The model under review builds one solid part; all positions refer to its coordinate system, in mm. Coordinates: 2 decimals unless noted, no trailing zeros. Order: outer loops, then holes, each group sorted by start corner. A loop starts at its lowest first (then second) coordinate and runs counter-clockwise, first axis right, second up. Notation, with made-up numbers: (61, 5.5) -> (111, 5.5) arc R24 ccw to (111, 26.5) -> close; hole circle Ø1 at (-36, -26.75). An arc over 180 degrees is marked (long way). Use one line per item in the form item = value.
from build123d import *

# Parameters (mm, degrees)
SKETCH1_W                     = 1
SKETCH1_H                     = 102
REVOLVE_THIN1_ANGLE           = 15
REVOLVE_THIN1_OTHER_WAY_ANGLE = 165
F_4_5_4_5_DIAMETER_HOLE1_D    = 4.5
CIRPATTERN1_COUNT             = 12
F_4_0_4_DIAMETER_HOLE1_D      = 4
CIRPATTERN2_COUNT             = 4
F_4_5_4_5_DIAMETER_HOLE2_D    = 4.5
CIRPATTERN3_COUNT             = 2
CIRPATTERN3_ANGLE             = 90
CUT_EXTRUDE1_DEPTH            = 2
CUT_EXTRUDE2_DEPTH            = 2
FILLET1_R                     = 1


with BuildPart() as part:
    # Sketch1 → Revolve-Thin1 (revolve)
    with BuildSketch(Plane(origin=(0, 0, 0), x_dir=(0, 0, -1), z_dir=(1, 0, 0))):
        with Locations((-0.5, 80)):
            Rectangle(SKETCH1_W, SKETCH1_H)
    revolve(axis=Axis((0, 0, 0), (0, 0, 1)), revolution_arc=REVOLVE_THIN1_ANGLE)

    # Sketch1 → Revolve-Thin1 other way (revolve)
    with BuildSketch(Plane(origin=(0, 0, 0), x_dir=(0, 0, -1), z_dir=(1, 0, 0))):
        with Locations((-0.5, 80)):
            Rectangle(SKETCH1_W, SKETCH1_H)
    revolve(axis=Axis((0, 0, 0), (0, 0, -1)), revolution_arc=REVOLVE_THIN1_OTHER_WAY_ANGLE)

    # Ø4.5 (4.5) Diameter Hole1 (through all)
    with Locations(Plane.XY.offset(1)):
        with Locations((62.125, 107.60365642)):
            f_4_5_4_5_diameter_hole1 = Hole(F_4_5_4_5_DIAMETER_HOLE1_D / 2)

    # CirPattern1: Ø4.5 (4.5) Diameter Hole1 ×12 about axis, 8 skipped
    cirpattern1_axis = Axis((0, 0, -80.9), (0, 0, 1))
    add([f_4_5_4_5_diameter_hole1.rotate(cirpattern1_axis, i * 360 / CIRPATTERN1_COUNT) for i in range(1, CIRPATTERN1_COUNT) if i not in (1, 2, 3, 4, 5, 6, 7, 10)], mode=Mode.SUBTRACT)

    # Ø4.0 (4) Diameter Hole1 (through all)
    with Locations(Plane.XY.offset(1)):
        with Locations((124.25, 0)):
            f_4_0_4_diameter_hole1 = Hole(F_4_0_4_DIAMETER_HOLE1_D / 2)

    # CirPattern2: Ø4.0 (4) Diameter Hole1 ×4 about axis, 2 skipped
    cirpattern2_axis = Axis((0, 0, -80.9), (0, 0, 1))
    add([f_4_0_4_diameter_hole1.rotate(cirpattern2_axis, i * 360 / CIRPATTERN2_COUNT) for i in range(1, CIRPATTERN2_COUNT) if i not in (2, 3)], mode=Mode.SUBTRACT)

    # Ø4.5 (4.5) Diameter Hole2 (through all)
    with Locations(Plane.XY.offset(1)):
        with Locations((87.858017562, 87.858017562)):
            f_4_5_4_5_diameter_hole2 = Hole(F_4_5_4_5_DIAMETER_HOLE2_D / 2)

    # CirPattern3: Ø4.5 (4.5) Diameter Hole2 ×2 about axis
    cirpattern3_axis = Axis((0, 0, -80.9), (0, 0, -1))
    for i in range(1, CIRPATTERN3_COUNT):
        add(f_4_5_4_5_diameter_hole2.rotate(cirpattern3_axis, i * CIRPATTERN3_ANGLE / (CIRPATTERN3_COUNT - 1)), mode=Mode.SUBTRACT)

    # Sketch12 → Cut-Extrude1 (cut, through all)
    with BuildSketch(Plane.XY.offset(1)):
        with BuildLine():
            Line((0.707106781, 126.371320344), (2.121320344, 124.957106781))
            ThreePointArc((2.121320344, 124.957106781), (2.121320344, 122.128679656), (-0.707106781, 122.128679656))
            Line((-0.707106781, 122.128679656), (-2.121320344, 123.542893219))
            ThreePointArc((-2.121320344, 123.542893219), (-2.121320344, 126.371320344), (0.707106781, 126.371320344))
        make_face()
    extrude(amount=-CUT_EXTRUDE1_DEPTH, mode=Mode.SUBTRACT)

    # Sketch13 → Cut-Extrude2 (cut, through all)
    with BuildSketch(Plane.XY.offset(1)):
        Polygon((-33.905294908, 126.536283244), (33.905294908, -126.536283244), (34.001887491, -126.510401339), (-33.808702326, 126.562165148), align=None)
    extrude(amount=-CUT_EXTRUDE2_DEPTH, mode=Mode.SUBTRACT)

    # Fillet1
    fillet1_edges = [part.edges().sort_by_distance(p)[0] for p in [
        (-7.409115101, 28.037564327, 0.5),
        (7.602300266, -27.985800518, 0.5),
        (34.001877612, -126.510364472, 0.5),
        (-33.808692447, 126.562128281, 0.5),
    ]]
    fillet(fillet1_edges, radius=FILLET1_R)


solid = part.part
Item 1: We need section A-A (z = 0.6). State how many separate pieces and enclosed holes the cut face has, plus the area to 3 significant figures.
Results found:
separate_pieces = 1
enclosed_holes = 8
area = 25,500 mm²
Item 2: Draft analysis for pull direction Y (two halves, no side actions). For faces 1 (the face through (50, 4, 0)), 2 (the face through (125.764, 36.665, 0.493)), 3 (the face through (27.844, 8.106, 0.493)), state which applies: released by +Y, released by -Y, zero draft, split by the parting line, or undercut.
Results found:
face_1 = zero draft
face_2 = split by the parting line
face_3 = undercut
Item 3: To check wall thickness, follow L1, parallel to Y at x = 109.5, z = 0.45; L2, parallel to Y at x = -1, z = 0.35; L3, parallel to X at y = 62, z = 0.55. State the ranges of each line that lie inside material, in increasing order. Write a range as from..to.
Results found:
L1 = -71.91..-63.34, -60.91..60.91, 63.34..71.91
L2 = 28.98..122.42, 126.94..131
L3 = -16.51..105.36, 109.85..115.4
Item 4: Clearance check with flat-ended pins moving along their axes: pin 1 (7 mm diameter, centred on x = 62.12, y = 107.6, fed in from +Z); pin 2 (3.5 mm diameter, centred on x = 107.6, y = 62.12, fed in from +Z). State where each tip first meets the part, or that it passes through.
Results found:
pin_1 = 1
pin_2 = through
Item 5: We need section C-C (y = -15). Write out the cut boundary in (x, z), plus the area to 3 significant figures.
Results found:
outline = (24.82, 0) -> (130.14, 0) -> (130.14, 1) -> (24.82, 1) -> close
area = 105 mm²
Item 6: We need section B-B (x = -11). Write out the cut boundary in (y, z).
Results found:
outline = (41.44, 0) -> (130.54, 0) -> (130.54, 1) -> (41.44, 1) -> close
